Here's how the part is built. I have some questions about the finished solid (model axes, mm). Round coordinates to 2 decimals unless told otherwise and drop trailing zeros. Write each loop counter-clockwise with the first axis right and the second up, starting at its lowest first coordinate (ties: lowest second). Pieces come first, ordered by that corner, then holes. Notation, with made-up numbers: (11, 33) - (38, 33) arc R26 ccw to (38, 56) - close; hole circle Ø4 at (43.5, 84.5). An arc over 180 degrees is marked (long way). Use one line per item in the form item = value. Start each with the question number.
1. I want a section at C-C, the plane y = 0.5. List the corners of the cut face in (x, z) for me, plus the area to 3 significant figures.
2. Will these pins go through, and if not, where does the flat tip stop? pin 1 (2.5 mm diameter, centred on x = 1, z = 20, fed in from -Y); pin 2 (1.5 mm diameter, centred on x = 2, z = 20.5, fed in from +Y).
3. If I drill on line 1 along Z through (x, y) = (15.5, 0.35); line 2 along Y through (x, z) = (-15.5, 14.5); line 3 along Y through (x, z) = (1.5, -16), over which ranges is the centre line in solid material (lowest first)?
4. I want a section at D-D, the plane x = -8. List the corners of the cut face in (y, z) for me, plus the area to 3 significant figures.
5. I want a section at B-B, the plane z = 17.5. List the corners of the cut face in (x, y) for me.
6. I want a section at A-A, the plane x = 3. List the corners of the cut face in (y, z) for me.
```python
from build123d import *

# Parameters (mm, degrees)
SKETCH_1_W      = 60.5
SKETCH_1_H      = 37
EXTRUDE_1_DEPTH = 2.1
SKETCH_2_W      = 57.01
SKETCH_2_H      = 29.49
EXTRUDE_2_DEPTH = 0.1
SKETCH_5_W      = 55.01
SKETCH_5_H      = 27.49
EXTRUDE_4_DEPTH = 0.1
SKETCH_3_W      = 12.5
SKETCH_3_H      = 0.3
EXTRUDE_3_DEPTH = 3


with BuildPart() as part:
    # 草图1 → 凸台-拉伸1 (new body)
    with BuildSketch(Plane(origin=(0, 0, 0), x_dir=(1, 0, 0), z_dir=(0, 1, 0))):
        Rectangle(SKETCH_1_W, SKETCH_1_H)
    extrude(amount=EXTRUDE_1_DEPTH)

    # 草图2 → 凸台-拉伸2 (add)
    with BuildSketch(Plane(origin=(0, 2.1, 0), x_dir=(1, 0, 0), z_dir=(0, 1, 0))):
        with Locations((0.005, 1.755)):
            Rectangle(SKETCH_2_W, SKETCH_2_H)
    extrude(amount=EXTRUDE_2_DEPTH)

    # 草图5 → 凸台-拉伸4 (add)
    with BuildSketch(Plane(origin=(0, 2.2, 0), x_dir=(1, 0, 0), z_dir=(0, 1, 0))):
        with Locations((0.005, 1.755)):
            Rectangle(SKETCH_5_W, SKETCH_5_H)
    extrude(amount=EXTRUDE_4_DEPTH)

    # 草图3 → 凸台-拉伸3 (add)
    with BuildSketch(Plane.XY.offset(18.5)):
        with Locations((0, 1.031860601)):
            Rectangle(SKETCH_3_W, SKETCH_3_H)
    extrude(amount=EXTRUDE_3_DEPTH)


solid = part.part
```
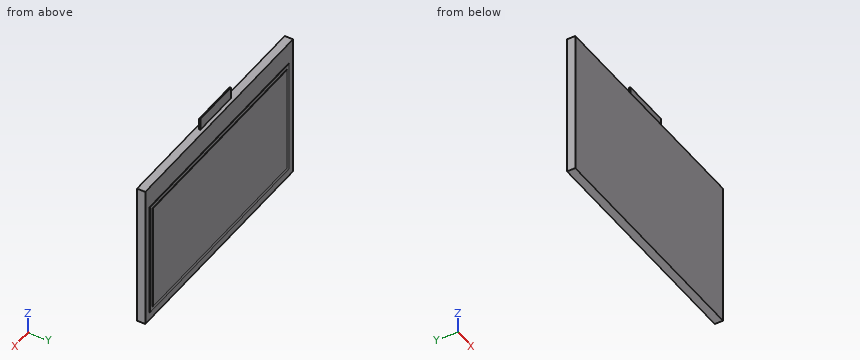
Model answer:
q1.outline = (-30.25, -18.5) - (30.25, -18.5) - (30.25, 18.5) - (-30.25, 18.5) - close
q1.area = 2,240 mm2
q2.pin_1 = 0.88
q2.pin_2 = 1.18
q3.line_1 = -18.5 to 18.5
q3.line_2 = 0 to 2.1
q3.line_3 = 0 to 2.2
q4.outline = (0, -18.5) - (2.1, -18.5) - (2.1, -16.5) - (2.2, -16.5) - (2.2, -15.5) - (2.3, -15.5) - (2.3, 11.99) - (2.2, 11.99) - (2.2, 12.99) - (2.1, 12.99) - (2.1, 18.5) - (0, 18.5) - close
q4.area = 83.4 mm2
q5.outline = (-30.25, 0) - (30.25, 0) - (30.25, 2.1) - (-30.25, 2.1) - close
q6.outline = (0, -18.5) - (2.1, -18.5) - (2.1, -16.5) - (2.2, -16.5) - (2.2, -15.5) - (2.3, -15.5) - (2.3, 11.99) - (2.2, 11.99) - (2.2, 12.99) - (2.1, 12.99) - (2.1, 18.5) - (1.18, 18.5) - (1.18, 21.5) - (0.88, 21.5) - (0.88, 18.5) - (0, 18.5) - close
